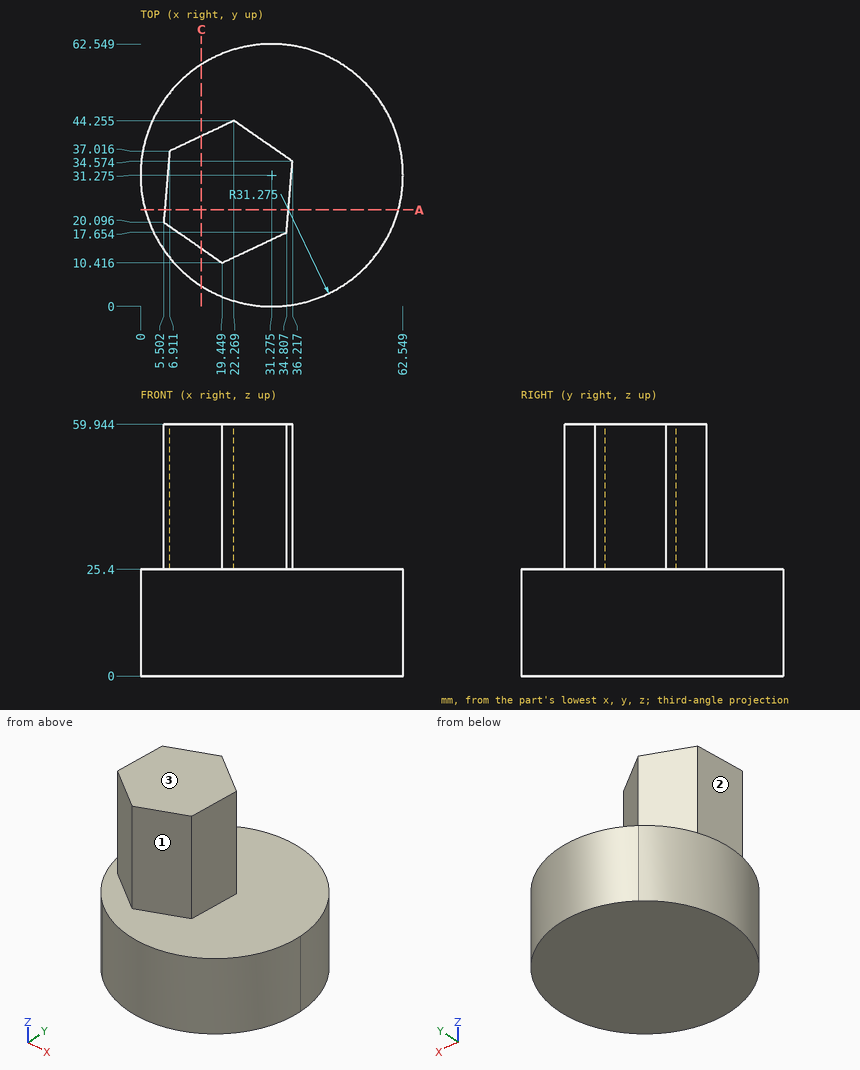
The drawing under review shows one solid part. Ordinate dimensions are in mm from its lowest x, y, z. A direction names the side the tool comes from. Coordinates: 2 decimals unless noted, no trailing zeros. Write each loop counter-clockwise with the first axis right and the second up, starting at its lowest first coordinate (ties: lowest second). Pieces come first, ordered by that corner, then holes. Notation, with made-up numbers: M -28.75,21 L 21.25,21 A18 ccw 21.25,52 Z; hole C 31.5,-28.5 d10. An arc over 180 degrees is marked long. Answer as a JSON object with one key per item and string values.
Item 1: Add section A-A, the plane y = 23. Give the boundary of the cut face in (x, z) (1 decimal), and give its area (3 significant figures).
Outcome:
{"outline": "M 1.1,0 L 61.4,0 L 61.4,25.4 L 35.3,25.4 L 35.3,59.9 L 5.7,59.9 L 5.7,25.4 L 1.1,25.4 Z", "area": "2,550 mm²"}
Item 2: Insertion check: pin 1 Ø1 at (x, y) = (42.5, 45) entering from +Z; pin 2 Ø1.5 at (y, z) = (21.5, 34.5) entering from +X; pin 3 Ø10 at (x, z) = (36, 11) entering from +Y; pin 4 Ø10 at (x, z) = (54, 33.5) entering from +Y. Each pin has a flat end and moves straight along its axis. Give the tip position at first contact, or say it passes through.
Outcome:
{"pin 1": "z = 25.4", "pin 2": "x = 35.19", "pin 3": "y = 62.55", "pin 4": "through"}
Item 3: Add section C-C, the plane x = 14.5. Give the boundary of the cut face in (y, z).
Outcome:
{"outline": "M 4.88,0 L 57.67,0 L 57.67,25.4 L 40.59,25.4 L 40.59,59.94 L 13.85,59.94 L 13.85,25.4 L 4.88,25.4 Z"}
Item 4: Wall thickness on probe 1 along Z at (x, y) = (22, 56); probe 2 along X at (y, z) = (29.5, 26) (1 decimal); probe 3 along Y at (x, z) = (32, 47.5): over which ranges is each line inside the solid? List them lowest first.
Outcome:
{"probe 1": "0 to 25.4", "probe 2": "6.3 to 35.8", "probe 3": "16.33 to 37.5"}
Item 5: Machinability: for the marked faces 1, 2 and 3, which of the approach directions +Z, -Z, +X, -X, +Y, -Y give a long, thin tool a straight path to every point of the face, cutting with its end or side? Answer none if there is none.
Outcome:
{"face 1": "+Z, +X, -Y", "face 2": "+Z, -X, +Y", "face 3": "+Z, +X, -X, +Y, -Y"}
